Geometry: final body of the model. Coordinates: model frame, mm. Face numbers are marked on the shaded views. A direction names the side the tool comes from. Give positions to 0.01 mm unless a question says otherwise; leave off trailing zeros. Write each loop counter-clockwise with the first axis right and the second up, starting at its lowest first coordinate (ties: lowest second). Pieces come first, ordered by that corner, then holes. Notation, with made-up numbers: (-22.75, 9.25) -> (-0.75, 9.25) arc R18 ccw to (-0.75, 29.25) -> close; hole circle Ø2 at (85.5, 69.25). An arc over 180 degrees is marked (long way). Answer in a Markdown table with one row per item. Add a question column.
Item 1: Material intervals for probe 1 along Y at (x, z) = (-9.5, 14.25); probe 2 along X at (y, z) = (19.25, 1); probe 3 along X at (y, z) = (1.25, 1.5), sorted ascending. Write a range as from..to.
Item 2: Access query for the marked faces 1, 2 and 3. Directions: +Z, -Z, +X, -X, +Y, -Y. A direction counts if a zero-diameter tool reaches every point of the face in a straight line with its end or side. Return the directions, or none.
Item 3: Section query D-D on z = 8. State how many separate pieces and enclosed holes the cut face has, plus the area to 3 significant figures.
Item 4: First-contact query: P1, Ø8, axis at y = 6.5, z = 4.5, coming from the -X side; P2, Ø11, axis at x = -15.5, z = 13.5, coming from the +Y side; P3, Ø6, axis at y = 15, z = 9, coming from the -X side. Flat tips, straight axial feed; report the tip coordinate or a pass-through.
Item 5: Section query B-B on x = -16. Output: boundary loops of the cut face in (y, z), plus the area to 3 significant figures.
Item 6: Draft query along X for the marked faces 4, 5 and 6. Return one class per face: +X half, -X half, draft (parallel to the pull), parting line (faces both ways), or undercut.
Autodesk Inventor part; units mm, degrees
ref_plane "YZ Plane" through (0, 0, 0) normal (1, 0, 0) x (0, 1, 0)
ref_plane "XZ Plane" through (0, 0, 0) normal (0, 1, 0) x (-1, 0, 0)
ref_plane "XY Plane" through (0, 0, 0) normal (0, 0, 1) x (1, 0, 0)
sketch "스케치1" plane through (0, 0, 0) normal (0, 0, 1) x (1, 0, 0)
  point P0 (0, 0)
sketch "스케치2" plane through (0, 0, 0) normal (0, 0, 1) x (1, 0, 0)
  point P0 (0, 0)
sketch "스케치3" plane through (0, 0, 0) normal (0, 0, 1) x (1, 0, 0)
  point P0 (0, 0)
sketch "스케치4" plane through (0, 0, 0) normal (0, 0, 1) x (1, 0, 0)
  line L0 (0, 0) -> (-38, 0)
  line L1 (-38, 0) -> (-38, 9)
  line L2 (-38, 9) -> (-8, 9)
  line L3 (-8, 9) -> (-8, 23)
  line L4 (-8, 23) -> (0, 23)
  line L5 (0, 23) -> (0, 0)
  dimension "d2" = 38
  dimension "d3" = 9
  dimension "d6" = 8
  dimension "d7" = 23
sketch "스케치5" plane through (0, 0, 0) normal (0, 0, 1) x (1, 0, 0)
  point P0 (0, 0)
extrude "돌출1" add sketch "스케치4" along normal blind 20
sketch "스케치6" plane through (-38, 9, 0) normal (0, 1, 0) x (1, 0, 0)
  point P0 (38, 0)
sketch "스케치7" plane through (-38, 9, 0) normal (0, 1, 0) x (1, 0, 0)
  line L0 (30, 0) -> (30, -20)
  line L1 (30, -14) -> (10, -14)
  line L2 (10, -14) -> (10, -6)
  line L3 (10, -6) -> (30, -6)
  line L4 (30, -6) -> (30, -14)
  line L5 (30, -20) -> (0, -20)
  line L6 (30, -6) -> (30, -14)
  line L7 (30, -6) -> (30, -14)
  line L8 (30, -14) -> (30, -6)
  line L9 (30, -14) -> (30, -6)
  point P0 (38, 0)
  dimension "d10" = 20
  dimension "d11" = 8
  dimension "d12" = 6
extrude "돌출2" cut sketch "스케치7" against normal blind 10
fillet "모깎기1" radius 10 2 edges at (-38, 4.5, 20) (-38, 4.5, 0)
fillet "모깎기2" radius 6 2 edges at (-4, 23, 20) (-4, 23, 0)
sketch "스케치8" plane through (-8, 0, 6) normal (-1, 0, 0) x (0, 0, 1)
  point P0 (-6, 0)
sketch "스케치9" plane through (-8, 0, 6) normal (-1, 0, 0) x (0, 0, 1)
  point P0 (-6, 0)
sketch "스케치10" plane through (-8, 0, 6) normal (-1, 0, 0) x (0, 0, 1)
  line L0 (0, 9) -> (0, 0)
  line L1 (8, 9) -> (8, 0)
  line L2 (0, 9) -> (8, 9)
  line L3 (-6, 9) -> (14, 9)
  line L4 (8, 9) -> (14, 9)
  line L5 (0, 9) -> (0, 0)
  point P0 (-6, 0)
sketch "스케치11" plane through (-8, 0, 6) normal (-1, 0, 0) x (0, 0, 1)
  line L0 (8, 9) -> (0, 9)
  line L1 (-6, 9) -> (0, 9)
  line L2 (0, 9) -> (-6, 9)
  point P0 (-6, 0)
sketch "스케치12" plane through (-8, 0, 6) normal (-1, 0, 0) x (0, 0, 1)
  line L0 (0, 17) -> (8, 17) construction
  line L1 (0, 14) -> (8, 14)
  line L2 (8, 20) -> (0, 20)
  arc A0 (0, 20) -> (0, 14) centre (0, 17) ccw
  arc A1 (8, 14) -> (8, 20) centre (8, 17) ccw
  line L3 (-6, 17) -> (-6, 9)
  line L4 (14, 0) -> (-6, 0)
  point P0 (4, 17)
  dimension "d18" = 8
  dimension "d19" = 6
  dimension "d20" = 10
  dimension "d21" = 17
sketch "스케치13" plane through (-8, 0, 6) normal (-1, 0, 0) x (0, 0, 1)
  point P0 (-6, 0)
extrude "돌출3" cut sketch "스케치12" against normal blind 10
fillet "모깎기3" radius 3 3 edges at (-35.0711, 9, 17.0711) (-18.0001, 9, 20) (-18.0001, 9, 0)
chamfer "모따기1" distance 5 angle 45 1 edges at (0, 0, 10)
properties part number "01_01"
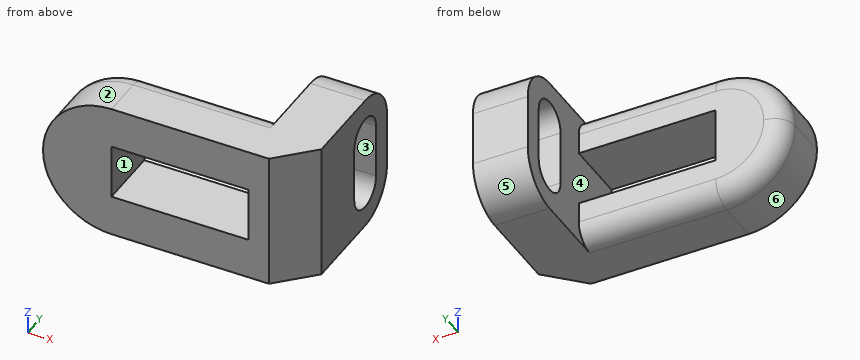
Findings below:
| question | item | result |
|---|---|---|
| 1 | probe 1 | y = 0..9 |
| 1 | probe 2 | x = -8..0 |
| 1 | probe 3 | x = -33.27..-3.75 |
| 2 | face 1 | +Y, -Y |
| 2 | face 2 | +Z, -X, +Y, -Y |
| 2 | face 3 | +X, -X |
| 3 | separate pieces | 3 |
| 3 | enclosed holes | 0 |
| 3 | area | 210 mm^2 |
| 4 | P1 | stops at x = -37.88 |
| 4 | P2 | stops at y = 9 |
| 4 | P3 | stops at x = -8 |
| 5 | outline | (0, 0) -> (6, 0) arc R3 ccw to (9, 3) -> (9, 6) -> (0, 6) -> close; (0, 14) -> (9, 14) -> (9, 17) arc R3 ccw to (6, 20) -> (0, 20) -> close |
| 5 | area | 104 mm^2 |
| 6 | face 4 | undercut |
| 6 | face 5 | draft |
| 6 | face 6 | -X half |
